```python
from build123d import *

# Parameters (mm, degrees)
SKETCH1_W               = 72.39
SKETCH1_H               = 12.7
BOSS_EXTRUDE1_DEPTH     = 0.635
SKETCH2_W               = 40.64
SKETCH2_H               = 12.7
BOSS_EXTRUDE2_DEPTH     = 1.27
F_6_CLEARANCE_HOLE1_D   = 3.7973
F_8_CLEARANCE_HOLE1_D   = 4.4958
CUT_EXTRUDE6_DEPTH      = 1
CUT_EXTRUDE6_DEPTH_BACK = 10.16


with BuildPart() as part:
    # Sketch1 → Boss-Extrude1 (new body)
    with BuildSketch(Plane(origin=(0, 0, 0), x_dir=(1, 0, 0), z_dir=(0, 1, 0))):
        with Locations((36.195, -6.35)):
            Rectangle(SKETCH1_W, SKETCH1_H)
    extrude(amount=BOSS_EXTRUDE1_DEPTH)

    # Sketch2 → Boss-Extrude2 (add)
    with BuildSketch(Plane(origin=(0, 0.635, 0), x_dir=(1, 0, 0), z_dir=(0, 1, 0))):
        with Locations((20.32, -6.35)):
            Rectangle(SKETCH2_W, SKETCH2_H)
    extrude(amount=BOSS_EXTRUDE2_DEPTH)

    # #6 Clearance Hole1 (through all)
    with Locations(Plane(origin=(0, 0, 0), x_dir=(-1, 0, 0), z_dir=(0, -1, 0))):
        with Locations((-67.31, -6.35), (-57.15, -6.35)):
            Hole(F_6_CLEARANCE_HOLE1_D / 2)

    # #8 Clearance Hole1 (through all)
    with Locations(Plane(origin=(0, 0, 0), x_dir=(-1, 0, 0), z_dir=(0, -1, 0))):
        with Locations((-12.7, -3.81)):
            Hole(F_8_CLEARANCE_HOLE1_D / 2)

    # Sketch9 → Cut-Extrude6 (cut, two sides)
    with BuildSketch(Plane.ZY) as cut_extrude6_sk:
        Polygon((1.563293937, 0.508), (1.27, 0), (1.856587873, 0), align=None)
        Polygon((2.14988181, 0.508), (1.856587873, 0), (2.443175747, 0), align=None)
        Polygon((0.87988181, 0.508), (0.586587873, 0), (1.173175747, 0), align=None)
        Polygon((0.293293937, 0.508), (0, 0), (0.586587873, 0), align=None)
        Polygon((2.833293937, 0.508), (2.54, 0), (3.126587873, 0), align=None)
        Polygon((3.41988181, 0.508), (3.126587873, 0), (3.713175747, 0), align=None)
        Polygon((4.103293937, 0.508), (3.81, 0), (4.396587873, 0), align=None)
        Polygon((4.68988181, 0.508), (4.396587873, 0), (4.983175747, 0), align=None)
        Polygon((5.373293937, 0.508), (5.08, 0), (5.666587873, 0), align=None)
        Polygon((5.95988181, 0.508), (5.666587873, 0), (6.253175747, 0), align=None)
        Polygon((6.643293937, 0.508), (6.35, 0), (6.936587873, 0), align=None)
        Polygon((7.22988181, 0.508), (6.936587873, 0), (7.523175747, 0), align=None)
        Polygon((7.913293937, 0.508), (7.62, 0), (8.206587873, 0), align=None)
        Polygon((8.49988181, 0.508), (8.206587873, 0), (8.793175747, 0), align=None)
        Polygon((9.183293937, 0.508), (8.89, 0), (9.476587873, 0), align=None)
        Polygon((9.76988181, 0.508), (9.476587873, 0), (10.063175747, 0), align=None)
        Polygon((10.453293937, 0.508), (10.16, 0), (10.746587873, 0), align=None)
        Polygon((11.03988181, 0.508), (10.746587873, 0), (11.333175747, 0), align=None)
        Polygon((11.723293937, 0.508), (11.43, 0), (12.016587873, 0), align=None)
        Polygon((12.30988181, 0.508), (12.016587873, 0), (12.603175747, 0), align=None)
    extrude(amount=CUT_EXTRUDE6_DEPTH, mode=Mode.SUBTRACT)
    extrude(cut_extrude6_sk.sketch, amount=-CUT_EXTRUDE6_DEPTH_BACK, mode=Mode.SUBTRACT)


solid = part.part
```
Geometry: final body of the model. Coordinates: model frame, mm. A direction names the side the tool comes from. Round coordinates to 2 decimals unless told otherwise and drop trailing zeros. Order: outer loops, then holes, each group sorted by start corner. A loop starts at its lowest first (then second) coordinate and runs counter-clockwise, first axis right, second up. Notation, with made-up numbers: M 16,87.5 L 53,87.5 A13 cw 53,103.5 Z; hole C -39.75,58.25 d6. An arc over 180 degrees is marked long. Use one line per item in the form item = value. Start each with the question number.
Q1. Mould query, pull axis X, two halves, no side actions, for faces 1 (the face through (55.253, 0.322, 6.267)), 2 (the face through (69.12, 0.32, 5.78)), 3 (the face through (28, 1, 12.7)), 4 (the face through (40.64, 1, 6)). Classes: +X half, -X half, draft (parallel to the pull), parting line (faces both ways), or undercut.
Q2. Access query for faces 5 (the face through (20, 1.905, 6)), 6 (the face through (56, 0.635, 9)). Directions: +Z, -Z, +X, -X, +Y, -Y. A direction counts if a zero-diameter tool reaches every point of the face in a straight line with its end or side. Return the directions, or none.
Q3. Cut plane A-A (x = 57.15). Return loops of the section in (y, z) (3 decimals).
Q4. Pin query (flat end, axial travel): pin 1 Ø4.5 at (x, z) = (57.15, 6.35) entering from +Y (3 decimals). Return the tip coordinate at first contact, or that it passes through.
Q5. Cut plane C-C (x = 12.7). Return loops of the section in (y, z) (3 decimals).
Q6. Cut plane B-B (y = 1.6). Return loops of the section in (x, z).
Q7. Material intervals for line 1 (X direction, y = 1.15, z = 3.75); line 2 (Z direction, x = 57.15, y = 0.4); line 3 (Z direction, x = 12.7, y = 1.25), sorted ascending. Write a range as [from, to].
Geometry results:
q1.face_1 = undercut
q1.face_2 = undercut
q1.face_3 = draft
q1.face_4 = +X half
q2.face_5 = +Z, -Z, +X, -X, +Y
q2.face_6 = +Z, -Z, +X, +Y
q3.outline = M 0,0 L 0.635,0 L 0.635,4.451 L 0,4.451 Z; M 0,8.249 L 0.635,8.249 L 0.635,12.7 L 0,12.7 Z
q4.pin_1 = 0.635
q5.outline = M 0,0 L 1.905,0 L 1.905,1.562 L 0,1.562 Z; M 0,6.058 L 1.905,6.058 L 1.905,12.7 L 0,12.7 Z
q6.outline = M 0,0 L 40.64,0 L 40.64,12.7 L 0,12.7 Z; hole C 12.7,3.81 d4.5
q7.line_1 = [0, 10.45], [14.95, 40.64]
q7.line_2 = [0, 4.45], [8.25, 12.7]
q7.line_3 = [0, 1.56], [6.06, 12.7]
